Read the model definition and answer for the solid it produces. Units are mm, in the model's axes. Face numbers are marked on the shaded views. A direction names the side the tool comes from. Give positions to 0.01 mm unless a question says otherwise; leave off trailing zeros. Write each loop counter-clockwise with the first axis right and the second up, starting at its lowest first coordinate (ties: lowest second). Pieces come first, ordered by that corner, then holes. Notation, with made-up numbers: (20, 58.5) -> (59, 58.5) arc R20 cw to (59, 86.5) -> close; hole circle Ø4 at (-27.75, 72.25). An arc over 180 degrees is marked (long way). Write item = value, one per line.
from build123d import *

# Parameters (mm, degrees)
F1_DEPTH = 170


with BuildPart() as f1:
    # F0 (on Front) → F1 (new body)
    with BuildSketch(Plane.XZ):
        with BuildLine():
            Line((-10, -5.857864), (-10, 0))
            Line((-10, 0), (-12.5, 0))
            Line((-12.5, 0), (-12.5, -5.857864))
            ThreePointArc((-12.5, -5.857864), (-12.958759, -7.30124), (-14.166667, -8.214887))
            ThreePointArc((-14.166667, -8.214887), (-22.319982, -22.113775), (-10, -32.5))
            Line((-10, -32.5), (10, -32.5))
            ThreePointArc((10, -32.5), (22.319982, -22.113775), (14.166667, -8.214887))
            ThreePointArc((14.166667, -8.214887), (12.958759, -7.30124), (12.5, -5.857864))
            Line((12.5, -5.857864), (12.5, 0))
            Line((12.5, 0), (10, 0))
            Line((10, 0), (10, -5.857864))
            ThreePointArc((10, -5.857864), (10.917517, -8.744616), (13.333333, -10.57191))
            ThreePointArc((13.333333, -10.57191), (19.855986, -21.69102), (10, -30))
            Line((10, -30), (-10, -30))
            ThreePointArc((-10, -30), (-19.855986, -21.69102), (-13.333333, -10.57191))
            ThreePointArc((-13.333333, -10.57191), (-10.917517, -8.744616), (-10, -5.857864))
        make_face()
    extrude(amount=F1_DEPTH)


solid = f1.part
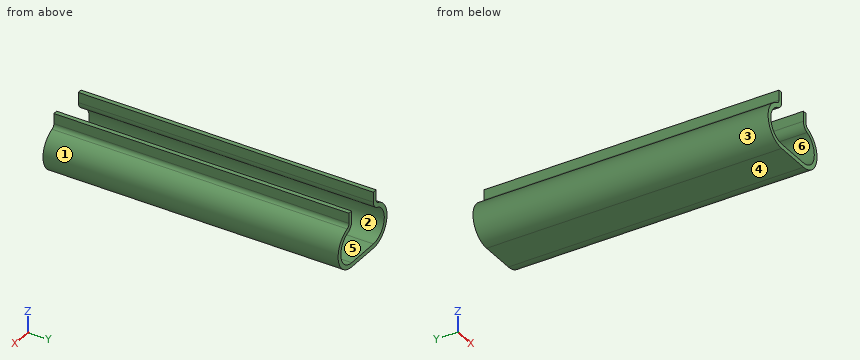
(1) A tool of negligible diameter and unlimited length cuts with its end or side. For the marked faces 4, 5 and 6, from which of +Z, -Z, +X, -X, +Y, -Y can it reach the whole face along a straight path? Write none if from no direction.
Checks:
face_4 = -Z, +X, -X, +Y, -Y
face_5 = +Z, +Y, -Y
face_6 = +Y, -Y
(2) For a pull along X with two mould halves and no side action, classify the marked faces 1, 2 and 3 as released by +X, released by -X, zero draft, split by the parting line, or undercut.
Checks:
face_1 = released by +X
face_2 = undercut
face_3 = released by -X
(3) Given P1, Ø6.5, axis at y = -53, z = -3.5, coming from the -X side; P2, Ø5, axis at x = 0, y = -56, coming from the +Z side; P3, Ø4, axis at x = 17.5, y = -34, coming from the +Z side (3 decimals), each flat-ended and moving along its own axis, determine where each tip first touches the part or whether it passes through.
Checks:
P1 = -12.66
P2 = -30
P3 = -8.775
(4) The part is cut by section D-D on x = -1. Determine the outline of the cut face in (y, z).
Checks:
outline = (-170, -32.5) -> (0, -32.5) -> (0, -30) -> (-170, -30) -> close
(5) The part is cut by section A-A on z = -14.5. Determine the outline of the cut face in (x, y).
Checks:
outline = (-21.22, -170) -> (-18.35, -170) -> (-18.35, 0) -> (-21.22, 0) -> close; (18.35, -170) -> (21.22, -170) -> (21.22, 0) -> (18.35, 0) -> close
(6) The part is cut by section C-C on x = -16.5. Determine the outline of the cut face in (y, z).
Checks:
outline = (-170, -30.68) -> (0, -30.68) -> (0, -27.6) -> (-170, -27.6) -> close; (-170, -12.4) -> (0, -12.4) -> (0, -9.32) -> (-170, -9.32) -> close
(7) The part is cut by section B-B on y = -49. Determine the outline of the cut face in (x, z), plus the area to 3 significant figures.
Checks:
outline = (-14.17, -8.21) arc R12.5 ccw to (-10, -32.5) -> (10, -32.5) arc R12.5 ccw to (14.17, -8.21) arc R2.5 cw to (12.5, -5.86) -> (12.5, 0) -> (10, 0) -> (10, -5.86) arc R5 ccw to (13.33, -10.57) arc R10 cw to (10, -30) -> (-10, -30) arc R10 cw to (-13.33, -10.57) arc R5 ccw to (-10, -5.86) -> (-10, 0) -> (-12.5, 0) -> (-12.5, -5.86) arc R2.5 cw to start
area = 260 mm²
(8) Consider L1, parallel to X at y = -117, z = -2; L2, parallel to X at y = -17, z = -20; L3, parallel to Z at x = 4, y = -49.5. Determine where each line is inside the solid, lowest interval first.
Checks:
L1 = -12.5 to -10, 10 to 12.5
L2 = -22.5 to -20, 20 to 22.5
L3 = -32.5 to -30
